Check sheet for the drawn part. Datum: minimum x, y, z corner. Units: mm. A direction names the side the tool comes from. Give positions to 0.01 mm unless a question says otherwise; leave off trailing zeros. Write each loop counter-clockwise with the first axis right and the second up, starting at its lowest first coordinate (ties: lowest second). Pieces come first, ordered by that corner, then holes. Notation, with made-up numbers: (-7.5, 51) -> (25.5, 51) arc R15 ccw to (25.5, 55) -> close; hole circle Ø4 at (61.5, 58.25). An arc over 180 degrees is marked (long way). Answer as CSV lines item,"result". Start each with the question number.
1) Mould release check, pull along Z, two halves, no side actions. Record for the marked faces 1, 2 and 3: released by +Z, released by -Z, zero draft, split by the parting line, or undercut.
2) Sectioned sample at A-A on y = 7.75. Record the cut outline in (x, z).
3) Material ranges on L1, parallel to X at y = 4, z = 12.25; L2, parallel to Z at x = 5.5, y = 8.5, recorded low to high.
4) Sectioned sample at B-B on z = 2.5. Record the cut outline in (x, y).
5) Tool access check on the marked faces 4 and 5. Record the directions out of +Z, -Z, +X, -X, +Y, -Y that give a thin tool (end or side, any length) a straight path to the whole face; none if there is none.
6) Gauge pin test, flat ends, axial feed: pin 1 Ø8 at (x, z) = (6.5, 13) entering from -Y; pin 2 Ø7 at (x, z) = (11.5, 12.5) entering from -Y. Record the tip position at first contact, or that the pin passes through.
7) Sectioned sample at D-D on x = 2. Record the cut outline in (y, z), and give its area (3 significant figures).
8) Sectioned sample at C-C on x = 9.5. Record the cut outline in (y, z).
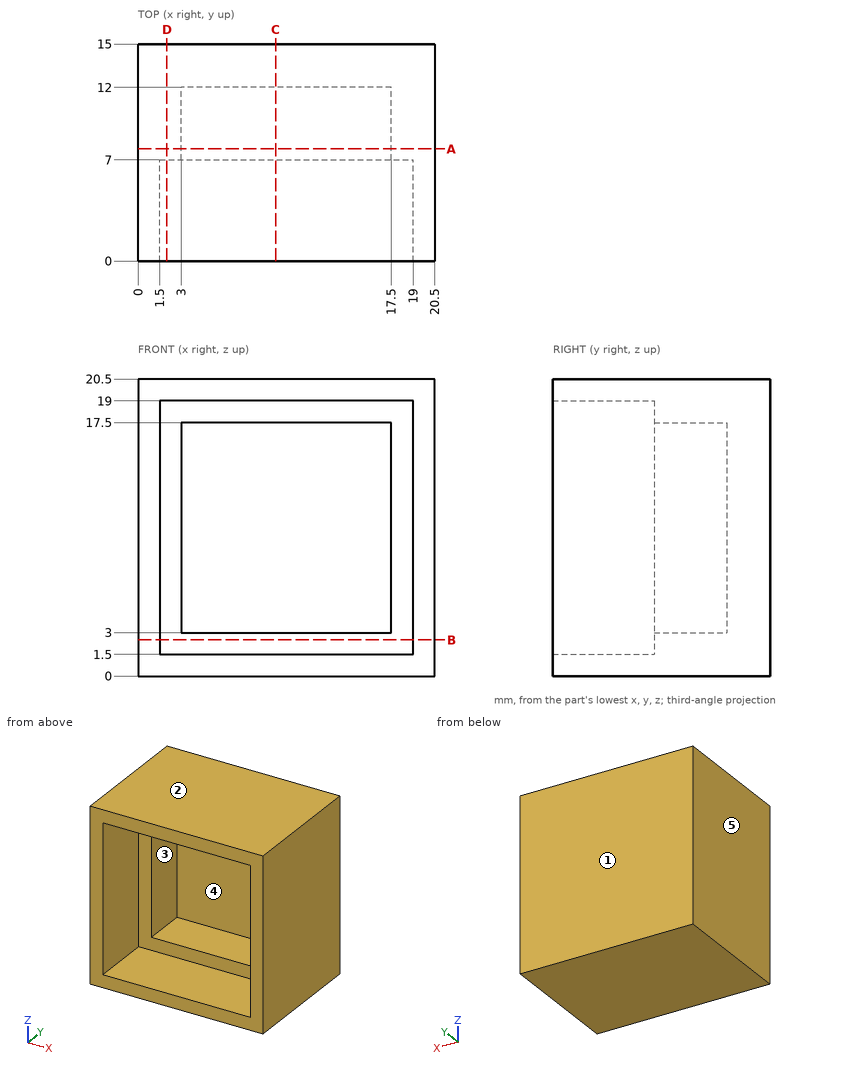
Ans:
1,face 1,"zero draft"
1,face 2,"released by +Z"
1,face 3,"undercut"
2,outline,"(0, 0) -> (20.5, 0) -> (20.5, 20.5) -> (0, 20.5) -> close; hole (3, 3) -> (17.5, 3) -> (17.5, 17.5) -> (3, 17.5) -> close"
3,L1,"x = 0 to 1.5, 19 to 20.5"
3,L2,"z = 0 to 3, 17.5 to 20.5"
4,outline,"(0, 0) -> (1.5, 0) -> (1.5, 7) -> (19, 7) -> (19, 0) -> (20.5, 0) -> (20.5, 15) -> (0, 15) -> close"
5,face 4,"-Y"
5,face 5,"+Z, -Z, -X, +Y, -Y"
6,pin 1,"stops at y = 7"
6,pin 2,"stops at y = 12"
7,outline,"(0, 0) -> (15, 0) -> (15, 20.5) -> (0, 20.5) -> (0, 19) -> (7, 19) -> (7, 1.5) -> (0, 1.5) -> close"
7,area,"185 mm²"
8,outline,"(0, 0) -> (15, 0) -> (15, 20.5) -> (0, 20.5) -> (0, 19) -> (7, 19) -> (7, 17.5) -> (12, 17.5) -> (12, 3) -> (7, 3) -> (7, 1.5) -> (0, 1.5) -> close"
